Can you work these out from the model? Positions are in its coordinate system, mm. Give positions to 0.01 mm unless a question says otherwise; leave off trailing zeros. Loops run counter-clockwise (first coordinate to the right, second up) from the corner with the lowest first, then second, coordinate; pieces in that order, holes last. Notation, with made-up numbers: M -39,30.5 L 17,30.5 A29 cw 17,59.5 Z; hole C 64.25,-25.75 d4. An arc over 180 degrees is marked long. Answer as a JSON object with one key per item and string values.
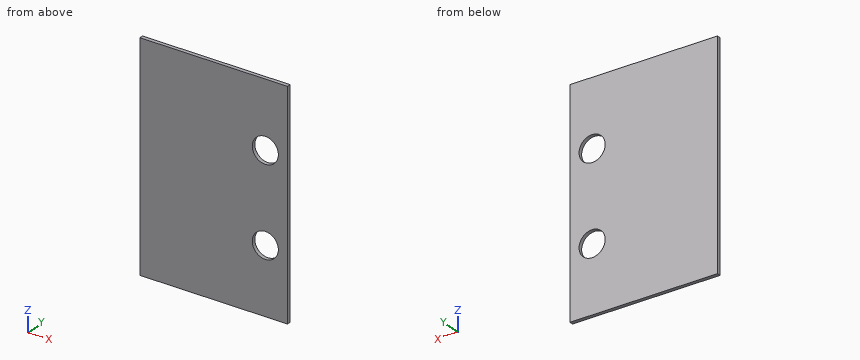
Autodesk Inventor part; units mm, degrees
ref_plane "YZ Plane" through (0, 0, 0) normal (1, 0, 0) x (0, 1, 0)
ref_plane "XZ Plane" through (0, 0, 0) normal (0, 1, 0) x (-1, 0, 0)
ref_plane "XY Plane" through (0, 0, 0) normal (0, 0, 1) x (1, 0, 0)
sketch "Sketch1" plane through (0, 0, 0) normal (0, 1, 0) x (-1, 0, 0)
  line L0 (12.2137, 18.6426) -> (-13.1863, 18.6426)
  line L1 (-13.1863, 18.6426) -> (-13.1863, -19.4574)
  line L2 (-13.1863, -19.4574) -> (12.2137, -19.4574)
  line L3 (12.2137, -19.4574) -> (12.2137, 18.6426)
  point P0 (0, 0)
  dimension "d0" = 25.4
  dimension "d1" = 38.1
extrude "Extrusion1" add sketch "Sketch1" along normal blind 0.635
hole "Hole1" at (9.3763, 0.635, 7.2126) direction (0, -1, 0) diameter 4.4958 depth 0.635
hole "Hole5" at (9.3763, 0.635, -8.0274) direction (0, -1, 0) diameter 4.4958 depth 25.4
properties part number "Shielding side"
1) Suppose I cut it at B-B, the plane y = 0.4. Write out the boundary of the cut face in (x, z).
Answer list:
{"outline": "M -12.21,-19.46 L 13.19,-19.46 L 13.19,18.64 L -12.21,18.64 Z; hole C 9.38,-8.03 d4.5; hole C 9.38,7.21 d4.5"}
2) Please list where these lines run through material, in increasing order: line 1 along Z through (x, y) = (10.5, 0.4); line 2 along Z through (x, y) = (8, 0.4); line 3 along X through (y, z) = (0.25, -7.5). Write a range as from..to.
Answer list:
{"line 1": "-19.46..-9.97, -6.08..5.27, 9.16..18.64", "line 2": "-19.46..-9.8, -6.25..5.44, 8.99..18.64", "line 3": "-12.21..7.19, 11.56..13.19"}
3) Suppose I cut it at A-A, the plane x = 7.5. Write out the boundary of the cut face in (y, z) (3 decimals), and give its area (3 significant figures).
Answer list:
{"outline": "M 0,-19.457 L 0.635,-19.457 L 0.635,-9.265 L 0,-9.265 Z; M 0,-6.789 L 0.635,-6.789 L 0.635,5.975 L 0,5.975 Z; M 0,8.451 L 0.635,8.451 L 0.635,18.643 L 0,18.643 Z", "area": "21.0 mm^2"}
